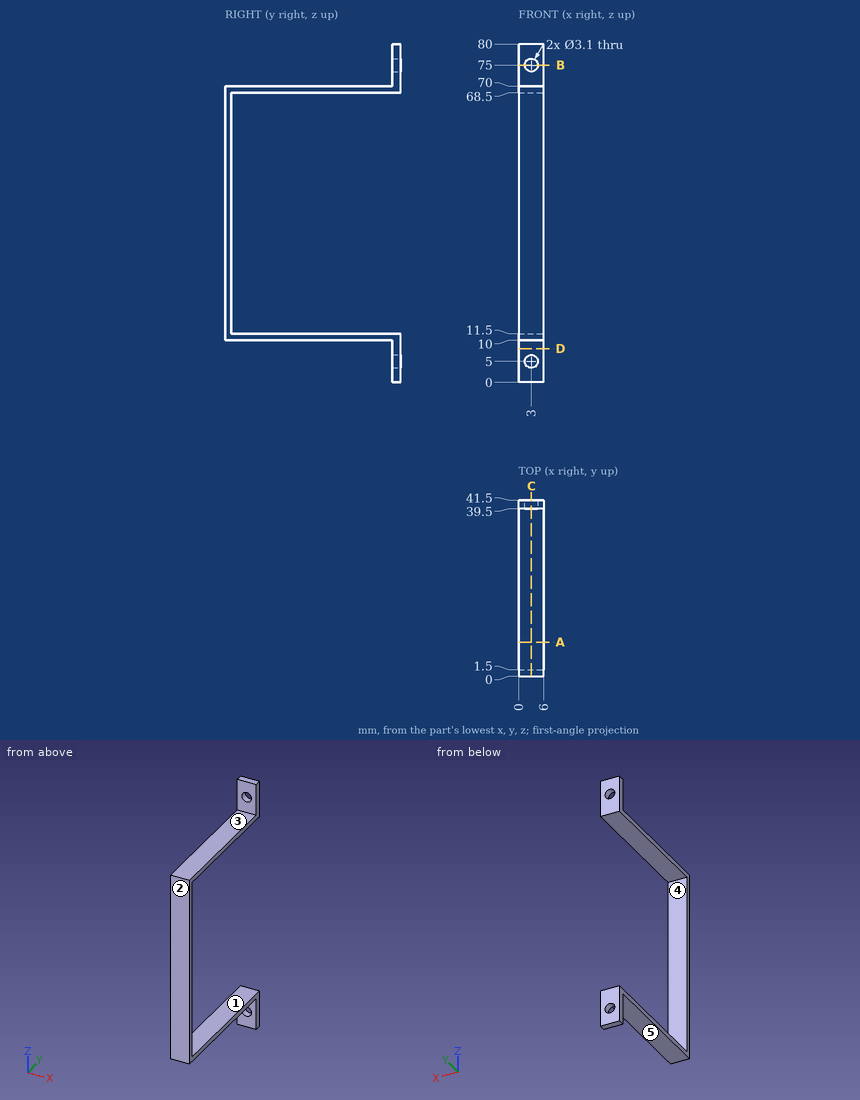
Input: dimensioned drawing with shaded views. Units: mm. Origin: part minimum x, y, z. A direction names the side the tool comes from. Coordinates: 2 decimals unless noted, no trailing zeros. Order: outer loops, then holes, each group sorted by start corner. A loop starts at its lowest first (then second) coordinate and runs counter-clockwise, first axis right, second up.
Item 1: Section query C-C (x = 3). Output: boundary loops of the cut face in (y, z), then the cut area to 3 significant figures.
Answer:
outline: (0, 10) - (39.5, 10) - (39.5, 6.55) - (41.5, 6.55) - (41.5, 11.5) - (1.5, 11.5) - (1.5, 68.5) - (41.5, 68.5) - (41.5, 73.45) - (39.5, 73.45) - (39.5, 70) - (0, 70) - close; (39.5, 0) - (41.5, 0) - (41.5, 3.45) - (39.5, 3.45) - close; (39.5, 76.55) - (41.5, 76.55) - (41.5, 80) - (39.5, 80) - close
area: 238 mm2
Item 2: Section query B-B (z = 75). Output: boundary loops of the cut face in (x, y), then the cut area to 3 significant figures.
Answer:
outline: (0, 39.5) - (1.45, 39.5) - (1.45, 41.5) - (0, 41.5) - close; (4.55, 39.5) - (6, 39.5) - (6, 41.5) - (4.55, 41.5) - close
area: 5.80 mm2
Item 3: Contact query for flat-ended pins moving along their axis: P1, Ø3, axis at x = 5, y = 25.5, coming from the +Z side; P2, Ø2, axis at x = 1.5, y = 28.5, coming from the -Z side; P3, Ø1.8, axis at x = 3, z = 77, coming from the -Y side; P4, Ø5, axis at y = 35.5, z = 70.5, coming from the +X side. Output: stop coordinate, or through.
Answer:
P1: stops at z = 70
P2: stops at z = 10
P3: stops at y = 39.5
P4: stops at x = 6
Item 4: Access query for the marked faces 4 and 5. Directions: +Z, -Z, +X, -X, +Y, -Y. A direction counts if a zero-diameter tool reaches every point of the face in a straight line with its end or side. Return the directions, or none.
Answer:
face 4: +X, -X, +Y
face 5: -Z, +X, -X, -Y
Item 5: Section query A-A (y = 8). Output: boundary loops of the cut face in (x, z), then the cut area to 3 significant figures.
Answer:
outline: (0, 10) - (6, 10) - (6, 11.5) - (0, 11.5) - close; (0, 68.5) - (6, 68.5) - (6, 70) - (0, 70) - close
area: 18.0 mm2
Item 6: Material intervals for line 1 along Z through (x, y) = (3, 40.2); line 2 along Z through (x, y) = (2.8, 38.5); line 3 along X through (y, z) = (40.7, 5), sorted ascending.
Answer:
line 1: z = 0 to 3.45, 6.55 to 11.5, 68.5 to 73.45, 76.55 to 80
line 2: z = 10 to 11.5, 68.5 to 70
line 3: x = 0 to 1.45, 4.55 to 6
Item 7: Draft query along Z for the marked faces 1, 2 and 3. Return one class per face: released by +Z, released by -Z, zero draft, split by the parting line, or undercut.
Answer:
face 1: undercut
face 2: zero draft
face 3: released by +Z
Item 8: Section query D-D (z = 8). Output: boundary loops of the cut face in (x, y).
Answer:
outline: (0, 39.5) - (6, 39.5) - (6, 41.5) - (0, 41.5) - close
